from build123d import *

# Parameters (mm, degrees)
SKETCH1_R           = 25
BOSS_EXTRUDE3_DEPTH = 5
FILLET3_R           = 2


with BuildPart() as part:
    # Sketch1 → Boss-Extrude3 (new body)
    with BuildSketch(Plane.XY):
        Circle(SKETCH1_R)
        with BuildLine():
            Line((-16.5, -14.028532992), (-18.42121658, -12.919318082))
            ThreePointArc((-18.42121658, -12.919318082), (-19.545793828, -11.145041212), (-20.5, -9.273618495))
            Line((-20.5, -9.273618495), (-20.5, -7.100329762))
            Line((-20.5, -7.100329762), (-16.5, -4.790928685))
            Line((-16.5, -4.790928685), (-12.5, -7.100329762))
            Line((-12.5, -7.100329762), (-12.5, -11.719131915))
            Line((-12.5, -11.719131915), (-16.5, -14.028532992))
        make_face(mode=Mode.SUBTRACT)
        with BuildLine():
            Line((-15, -16.770509831), (-15, -16.626609203))
            Line((-15, -16.626609203), (-11, -14.317208127))
            Line((-11, -14.317208127), (-7, -16.626609203))
            Line((-7, -16.626609203), (-7, -21.245411357))
            Line((-7, -21.245411357), (-7.1518668, -21.333091695))
            ThreePointArc((-7.1518668, -21.333091695), (-11.308429997, -19.451720001), (-15, -16.770509831))
        make_face(mode=Mode.SUBTRACT)
        with BuildLine():
            Line((-22, -4.618802154), (-22.023687548, -4.605126141))
            ThreePointArc((-22.023687548, -4.605126141), (-22.5, 0), (-22.023687548, 4.605126141))
            Line((-22.023687548, 4.605126141), (-22, 4.618802154))
            Line((-22, 4.618802154), (-18, 2.309401077))
            Line((-18, 2.309401077), (-18, -2.309401077))
            Line((-18, -2.309401077), (-22, -4.618802154))
        make_face(mode=Mode.SUBTRACT)
        Polygon((-1.5, -11.719131915), (-5.5, -14.028532992), (-9.5, -11.719131915), (-9.5, -7.100329762), (-5.5, -4.790928685), (-1.5, -7.100329762), align=None, mode=Mode.SUBTRACT)
        Polygon((-7, -2.309401077), (-11, -4.618802154), (-15, -2.309401077), (-15, 2.309401077), (-11, 4.618802154), (-7, 2.309401077), align=None, mode=Mode.SUBTRACT)
        with BuildLine():
            Line((4, -21.245411357), (1.977849369, -22.412900568))
            ThreePointArc((1.977849369, -22.412900568), (0, -22.5), (-1.977849369, -22.412900568))
            Line((-1.977849369, -22.412900568), (-4, -21.245411357))
            Line((-4, -21.245411357), (-4, -16.626609203))
            Line((-4, -16.626609203), (0, -14.317208127))
            Line((0, -14.317208127), (4, -16.626609203))
            Line((4, -16.626609203), (4, -21.245411357))
        make_face(mode=Mode.SUBTRACT)
        with BuildLine():
            Line((7.1518668, -21.333091695), (7, -21.245411357))
            Line((7, -21.245411357), (7, -16.626609203))
            Line((7, -16.626609203), (11, -14.317208127))
            Line((11, -14.317208127), (15, -16.626609203))
            Line((15, -16.626609203), (15, -16.770509831))
            ThreePointArc((15, -16.770509831), (11.308429997, -19.451720001), (7.1518668, -21.333091695))
        make_face(mode=Mode.SUBTRACT)
        Polygon((9.5, -11.719131915), (5.5, -14.028532992), (1.5, -11.719131915), (1.5, -7.100329762), (5.5, -4.790928685), (9.5, -7.100329762), align=None, mode=Mode.SUBTRACT)
        with BuildLine():
            Line((20.5, -7.100329762), (20.5, -9.273618496))
            ThreePointArc((20.5, -9.273618496), (19.545793828, -11.145041212), (18.42121658, -12.919318082))
            Line((18.42121658, -12.919318082), (16.5, -14.028532992))
            Line((16.5, -14.028532992), (12.5, -11.719131915))
            Line((12.5, -11.719131915), (12.5, -7.100329762))
            Line((12.5, -7.100329762), (16.5, -4.790928685))
            Line((16.5, -4.790928685), (20.5, -7.100329762))
        make_face(mode=Mode.SUBTRACT)
        with BuildLine():
            Line((-20.5, 7.216878365), (-20.5, 9.273618495))
            ThreePointArc((-20.5, 9.273618495), (-19.485571585, 11.25), (-18.281189202, 13.11671153))
            Line((-18.281189202, 13.11671153), (-16.5, 14.145081595))
            Line((-16.5, 14.145081595), (-12.5, 11.835680518))
            Line((-12.5, 11.835680518), (-12.5, 7.216878365))
            Line((-12.5, 7.216878365), (-16.5, 4.907477288))
            Line((-16.5, 4.907477288), (-20.5, 7.216878365))
        make_face(mode=Mode.SUBTRACT)
        Polygon((4, -2.309401077), (0, -4.618802154), (-4, -2.309401077), (-4, 2.309401077), (0, 4.618802154), (4, 2.309401077), align=None, mode=Mode.SUBTRACT)
        Polygon((-1.5, 7.216878365), (-5.5, 4.907477288), (-9.5, 7.216878365), (-9.5, 11.835680518), (-5.5, 14.145081595), (-1.5, 11.835680518), align=None, mode=Mode.SUBTRACT)
        with BuildLine():
            ThreePointArc((-15, 16.770509831), (-11.301438227, 19.455783048), (-7.136530526, 21.338227013))
            Line((-7.136530526, 21.338227013), (-7, 21.259401077))
            Line((-7, 21.259401077), (-7, 16.640598923))
            Line((-7, 16.640598923), (-11, 14.331197846))
            Line((-11, 14.331197846), (-15, 16.640598923))
            Line((-15, 16.640598923), (-15, 16.770509831))
        make_face(mode=Mode.SUBTRACT)
        with BuildLine():
            Line((-4, 21.259401077), (-2.006489815, 22.410354719))
            ThreePointArc((-2.006489815, 22.410354719), (0, 22.5), (2.006489815, 22.410354719))
            Line((2.006489815, 22.410354719), (4, 21.259401077))
            Line((4, 21.259401077), (4, 16.640598923))
            Line((4, 16.640598923), (0, 14.331197846))
            Line((0, 14.331197846), (-4, 16.640598923))
            Line((-4, 16.640598923), (-4, 21.259401077))
        make_face(mode=Mode.SUBTRACT)
        Polygon((15, -2.309401077), (11, -4.618802154), (7, -2.309401077), (7, 2.309401077), (11, 4.618802154), (15, 2.309401077), align=None, mode=Mode.SUBTRACT)
        Polygon((9.5, 7.216878365), (5.5, 4.907477288), (1.5, 7.216878365), (1.5, 11.835680518), (5.5, 14.145081595), (9.5, 11.835680518), align=None, mode=Mode.SUBTRACT)
        with BuildLine():
            Line((22.023687548, -4.605126141), (22, -4.618802154))
            Line((22, -4.618802154), (18, -2.309401077))
            Line((18, -2.309401077), (18, 2.309401077))
            Line((18, 2.309401077), (22, 4.618802154))
            Line((22, 4.618802154), (22.023687548, 4.605126141))
            ThreePointArc((22.023687548, 4.605126141), (22.5, 0), (22.023687548, -4.605126141))
        make_face(mode=Mode.SUBTRACT)
        with BuildLine():
            Line((20.5, 7.216878365), (16.5, 4.907477288))
            Line((16.5, 4.907477288), (12.5, 7.216878365))
            Line((12.5, 7.216878365), (12.5, 11.835680518))
            Line((12.5, 11.835680518), (16.5, 14.145081595))
            Line((16.5, 14.145081595), (18.281189202, 13.11671153))
            ThreePointArc((18.281189202, 13.11671153), (19.485571585, 11.25), (20.5, 9.273618496))
            Line((20.5, 9.273618496), (20.5, 7.216878365))
        make_face(mode=Mode.SUBTRACT)
        with BuildLine():
            ThreePointArc((7.136530526, 21.338227013), (11.301438227, 19.455783048), (15, 16.770509831))
            Line((15, 16.770509831), (15, 16.640598923))
            Line((15, 16.640598923), (11, 14.331197846))
            Line((11, 14.331197846), (7, 16.640598923))
            Line((7, 16.640598923), (7, 21.259401077))
            Line((7, 21.259401077), (7.136530526, 21.338227013))
        make_face(mode=Mode.SUBTRACT)
    extrude(amount=BOSS_EXTRUDE3_DEPTH)

    # Fillet3
    fillet3_edges = [part.edges().sort_by_distance(p)[0] for p in [
        (-25, 0, 0),
        (-25, 0, 5),
    ]]
    fillet(fillet3_edges, radius=FILLET3_R)


solid = part.part
For this review, take the finished solid that the model builds, in its own axes (mm). Give positions to 0.01 mm unless a question says otherwise; leave off trailing zeros. Order: outer loops, then holes, each group sorted by start corner. A loop starts at its lowest first (then second) coordinate and runs counter-clockwise, first axis right, second up. Notation, with made-up numbers: (11, -37) - (16, -37) arc R21 cw to (16, -15) - close; hole circle Ø4 at (14, 66.5). An arc over 180 degrees is marked (long way). Answer as a JSON object with one key per item and string values. Group by question number.
Item 1: Clearance check with flat-ended pins moving along their axes: pin 1 Ø2.5 at (y, z) = (19.5, 2) entering from -X; pin 2 Ø1.4 at (y, z) = (-19.5, 1.5) entering from +X; pin 3 Ø2.5 at (y, z) = (-8.5, 3.5) entering from -X; pin 4 Ø10 at (x, y) = (-2, 1.5) entering from -Z. State where each tip first meets the part, or that it passes through.
Item 2: Take a section at B-B on x = 19. Give the number of separate pieces and of enclosed holes in the cut face, and give its area (3 significant figures).
Item 3: Take a section at A-A on y = 0. Give the boundary of the cut face in (x, z).
Item 4: Draft analysis for pull direction X (two halves, no side actions). For faces 1 (the flat face through (0, -5, 5)), 2 (the flat face through (14.472, 12.974, 2.465)), state which applies: pulls with the +X half, pulls with the -X half, needs draft (parallel to the pull), parting line crosses it, or undercut.
Item 5: Wall thickness on line 1 along X through (y, z) = (13, 0.8); line 2 along X through (y, z) = (-10.5, 3.45); line 3 along X through (y, z) = (-18.5, 4.35): over which ranges is each line inside the solid? List them lowest first.
Reported:
{
 "1": {"pin 1": "x = -17.09", "pin 2": "x = 16.41", "pin 3": "x = -23.9", "pin 4": "z = 0"},
 "2": {"separate pieces": "4", "enclosed holes": "0", "area": "70.6 mm^2"},
 "3": {"outline": "(-25, 2) arc R2 ccw to (-23, 0) - (-22.5, 0) - (-22.5, 5) - (-23, 5) arc R2 ccw to (-25, 3) - close; (-18, 0) - (-15, 0) - (-15, 5) - (-18, 5) - close; (-7, 0) - (-4, 0) - (-4, 5) - (-7, 5) - close; (4, 0) - (7, 0) - (7, 5) - (4, 5) - close; (15, 0) - (18, 0) - (18, 5) - (15, 5) - close; (22.5, 0) - (23, 0) arc R2 ccw to (25, 2) - (25, 3) arc R2 ccw to (23, 5) - (22.5, 5) - close"},
 "4": {"face 1": "needs draft", "face 2": "undercut"},
 "5": {"line 1": "-20.88 to -18.36, -14.52 to -7.48, -3.52 to 3.52, 7.48 to 14.52, 18.36 to 20.88", "line 2": "-22.63 to -19.9, -12.5 to -9.5, -1.5 to 1.5, 9.5 to 12.5, 19.9 to 22.63", "line 3": "-16.03 to -12.81, -7 to -4, 4 to 7, 12.81 to 16.03"}
}
